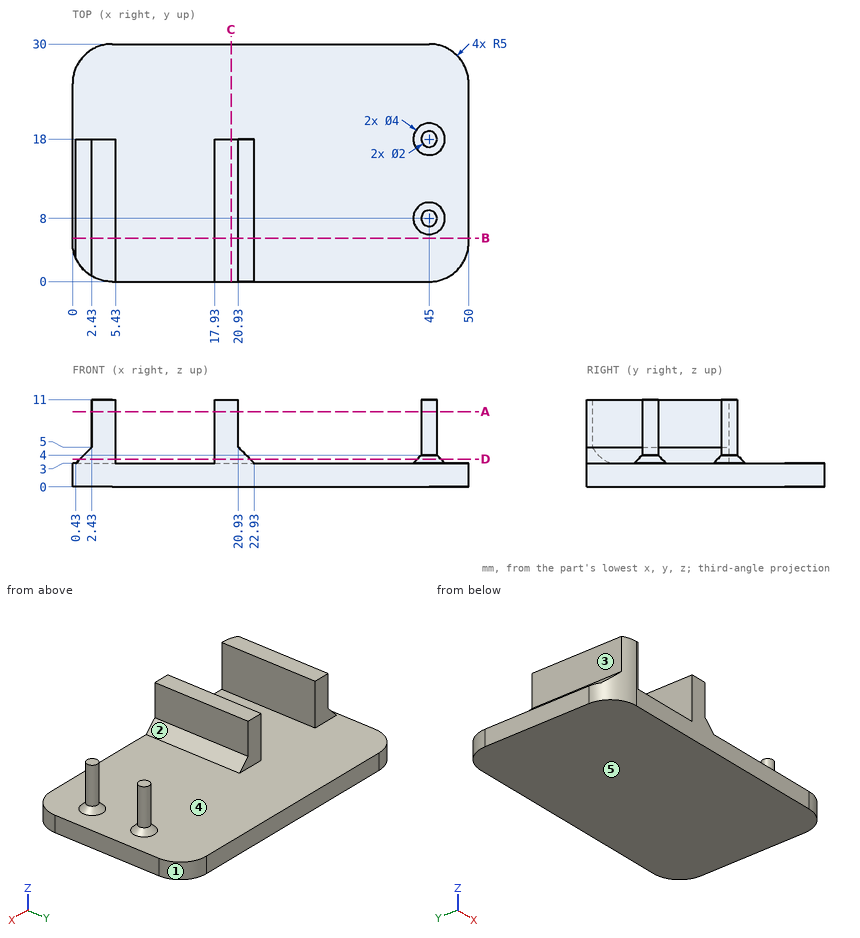
Input: dimensioned drawing with shaded views. Units: mm. Origin: part minimum x, y, z. A direction names the side the tool comes from. Coordinates: 2 decimals unless noted, no trailing zeros. Loops run counter-clockwise (first coordinate to the right, second up) from the corner with the lowest first, then second, coordinate; pieces in that order, holes last. Notation, with made-up numbers: M -35.5,10 L -21.5,10 A3 ccw -21.5,14 Z; hole C -40,69 d5. An arc over 180 degrees is marked long. One line per item, written item: value.
(1) Section C-C (x = 20). Output: boundary loops of the cut face in (y, z).
Filled in:
outline: M 0,0 L 30,0 L 30,3 L 18,3 L 18,11 L 0,11 Z
(2) Section D-D (z = 3.5). Output: boundary loops of the cut face in (x, y) (1 decimal).
Filled in:
outline: M 0.9,2.1 A5 ccw 5,0 L 5.4,0 L 5.4,18 L 0.9,18 Z; M 17.9,0 L 22.4,0 L 22.4,18 L 17.9,18 Z; C 45,8 d3; C 45,18 d3
(3) Pull-direction query (X, two-part tool) for the marked faces 3, 4 and 5; classes: +X half, -X half, draft (parallel to the pull), parting line (faces both ways), or undercut.
Filled in:
face 3: -X half
face 4: undercut
face 5: draft
(4) Line query: line 1 along X through (y, z) = (15, 10.75); line 2 along X through (y, z) = (7.5, 6.75) (1 decimal); line 3 along Y through (x, z) = (19, 4.75). Output: solid intervals per line, ascending. Write a range as from..to.
Filled in:
line 1: 2.43..5.43, 17.93..20.93
line 2: 2.4..5.4, 17.9..20.9, 44.1..45.9
line 3: 0..18
(5) Pin query (flat end, axial travel): pin 1 (15 mm diameter, centred on x = 32.5, y = 8.5, fed in from +Z); pin 2 (2.5 mm diameter, centred on y = 6.5, z = 8.5, fed in from +X); pin 3 (5 mm diameter, centred on y = 11, z = 7, fed in from -X). Return the tip coordinate at first contact, or that it passes through.
Filled in:
pin 1: z = 3
pin 2: x = 45.97
pin 3: x = 1.93
(6) Section A-A (z = 9.5). Output: boundary loops of the cut face in (x, y).
Filled in:
outline: M 2.43,0.71 A5 ccw 5,0 L 5.43,0 L 5.43,18 L 2.43,18 Z; M 17.93,0 L 20.93,0 L 20.93,18 L 17.93,18 Z; C 45,8 d2; C 45,18 d2
(7) Reachability of the marked faces 1 and 2 from +Z, -Z, +X, -X, +Y, -Y: full face, straight path, thin tool, end or side. Return the list, or none.
Filled in:
face 1: +Z, -Z, +X, +Y
face 2: +Z, +Y, -Y
(8) Section B-B (y = 5.5). Output: boundary loops of the cut face in (x, z).
Filled in:
outline: M 0,0 L 50,0 L 50,3 L 22.93,3 L 20.93,5 L 20.93,11 L 17.93,11 L 17.93,3 L 5.43,3 L 5.43,11 L 2.43,11 L 2.43,5 L 0.43,3 L 0,3 Z
